```python
from build123d import *

# Parameters (mm, degrees)
F0_W     = 25.4
F0_H     = 1.27
F1_DEPTH = 12.7
F2_R     = 2.54
F3_DEPTH = 1.271
F4_R     = 17.78
F5_DEPTH = 3.175
F6_R     = 6.35
F7_DEPTH = 6.351


with BuildPart() as f1:
    # F0 (on Front) → F1 (new body, symmetric)
    with BuildSketch(Plane.XZ):
        with Locations((12.7, 1.651)):
            Rectangle(F0_W, F0_H)
    extrude(amount=F1_DEPTH, both=True)

    # F2 (on face) → F3 (cut, through all)
    with BuildSketch(Plane(origin=(0, 0, 1.016), x_dir=(1, 0, 0), z_dir=(0, 0, -1))):
        with Locations((10.16, 8.300591)):
            Circle(F2_R)
        with Locations((10.16, -8.300591)):
            Circle(F2_R)
    extrude(amount=-F3_DEPTH, mode=Mode.SUBTRACT)

    # F4 (on Top) → F5 (join, symmetric)
    with BuildSketch(Plane.XY):
        with Locations((-11.176, 0)):
            Circle(F4_R)
    extrude(amount=F5_DEPTH, both=True)

    # F6 (on face) → F7 (cut, through all)
    with BuildSketch(Plane.XY.offset(3.175)):
        with Locations((-11.176, 0)):
            Circle(F6_R)
    extrude(amount=-F7_DEPTH, mode=Mode.SUBTRACT)


solid = f1.part
```
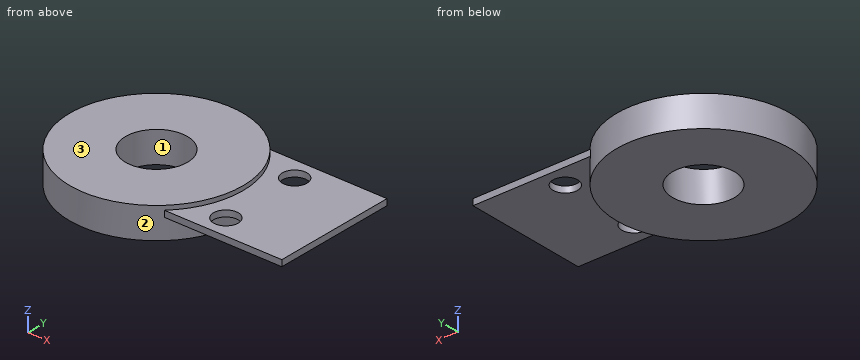
CAD build for the part. Positions are in the model's coordinates, mm. Face numbers are marked on the shaded views. Round coordinates to 2 decimals unless told otherwise and drop trailing zeros. Loops run counter-clockwise (first coordinate to the right, second up) from the corner with the lowest first, then second, coordinate; pieces in that order, holes last. Notation, with made-up numbers: M -34,81.5 L -9,81.5 A15 cw -9,95.5 Z; hole C 31.25,35.25 d3. An arc over 180 degrees is marked long. Use a Markdown table: item, result. Add a question column.
(1) Cut at D-D (y = -7.5). Give the cut face in (x, z) (3 decimals).
(2) Cut at B-B (y = 0). Give the cut face in (x, z) (3 decimals), and give its area (3 significant figures).
(3) Cut at C-C (x = -8.5). Give the cut face in (y, z) (3 decimals).
(4) Pull direction Y, two halves, no side cores. Call the marked faces 1, 2 and 3: +Y half, -Y half, draft (parallel to the pull), parting line (faces both ways), or undercut.
(5) Flat gauge pins, fed straight in: pin 1 (20.5 mm diameter, centred on x = -11.176, y = 0, fed in from -Z) (3 decimals); pin 2 (0.6 mm diameter, centred on x = 14, z = 2, fed in from -Y); pin 3 (1.5 mm diameter, centred on y = -6.5, z = -0.5, fed in from +X); pin 4 (2 mm diameter, centred on x = 15.5, y = -5.5, fed in from +Z). Where does each tip first touch, or does it go through?
(6) Cut at A-A (x = 10.16). Give the cut face in (y, z), and give its area (3 significant figures).
(7) Drill centre lines: line 1 (Y direction, x = 10.16, z = 1.9); line 2 (Y direction, x = -15, z = 0.75); line 3 (Z direction, x = 20, y = -10). Where is each one in solid material? Low to high.
Geometry says:
| question | item | result |
|---|---|---|
| 1 | outline | M -27.297,-3.175 L 4.945,-3.175 L 4.945,1.016 L 7.749,1.016 L 7.749,2.286 L 4.945,2.286 L 4.945,3.175 L -27.297,3.175 Z; M 12.571,1.016 L 25.4,1.016 L 25.4,2.286 L 12.571,2.286 Z |
| 2 | outline | M -28.956,-3.175 L -17.526,-3.175 L -17.526,3.175 L -28.956,3.175 Z; M -4.826,-3.175 L 6.604,-3.175 L 6.604,1.016 L 25.4,1.016 L 25.4,2.286 L 6.604,2.286 L 6.604,3.175 L -4.826,3.175 Z |
| 2 | area | 169 mm² |
| 3 | outline | M -17.577,-3.175 L -5.759,-3.175 L -5.759,3.175 L -17.577,3.175 Z; M 5.759,-3.175 L 17.577,-3.175 L 17.577,3.175 L 5.759,3.175 Z |
| 4 | face 1 | undercut |
| 4 | face 2 | parting line |
| 4 | face 3 | draft |
| 5 | pin 1 | stops at z = -3.175 |
| 5 | pin 2 | stops at y = -12.7 |
| 5 | pin 3 | stops at x = 5.65 |
| 5 | pin 4 | stops at z = 2.29 |
| 6 | outline | M -12.7,1.02 L -10.84,1.02 L -10.84,2.29 L -12.7,2.29 Z; M -5.76,1.02 L 5.76,1.02 L 5.76,2.29 L -5.76,2.29 Z; M 10.84,1.02 L 12.7,1.02 L 12.7,2.29 L 10.84,2.29 Z |
| 6 | area | 19.4 mm² |
| 7 | line 1 | y = -12.7 to -10.84, -5.76 to 5.76, 10.84 to 12.7 |
| 7 | line 2 | y = -17.36 to -5.07, 5.07 to 17.36 |
| 7 | line 3 | z = 1.02 to 2.29 |
